Geometry: final body of the model. Coordinates: model frame, mm. Give positions to 0.01 mm unless a question says otherwise; leave off trailing zeros. Write each loop counter-clockwise with the first axis right and the second up, starting at its lowest first coordinate (ties: lowest second). Pieces come first, ordered by that corner, then holes. Notation, with made-up numbers: M 49.25,-1 L 79.25,-1 A18 ccw 79.25,27 Z; hole C -12.75,15 d8. An arc over 180 degrees is marked long. Answer as a JSON object with one key per item and string values.
from build123d import *

# Parameters (mm, degrees)
ESQUISSE1_R        = 75
ESQUISSE1_R_2      = 0.8
ESQUISSE1_R_3      = 3
ESQUISSE1_R_4      = 2
BOSS_EXTRU_1_DEPTH = 10


with BuildPart() as part:
    # Esquisse1 → Boss.-Extru.1 (new body)
    with BuildSketch(Plane(origin=(0, 0, 0), x_dir=(1, 0, 0), z_dir=(0, 1, 0))):
        with Locations(Location((0, 0, 0), (0, 0, 270))):
            Circle(ESQUISSE1_R)
        with Locations(Location((0, -7.5, 0), (0, 0, 270))):
            Circle(ESQUISSE1_R_2, mode=Mode.SUBTRACT)
        with Locations(Location((-7.5, 0, 0), (0, 0, 270))):
            Circle(ESQUISSE1_R_2, mode=Mode.SUBTRACT)
        with Locations(Location((0, 7.5, 0), (0, 0, 270))):
            Circle(ESQUISSE1_R_2, mode=Mode.SUBTRACT)
        with Locations(Location((7.5, 0, 0), (0, 0, 270))):
            Circle(ESQUISSE1_R_2, mode=Mode.SUBTRACT)
        with Locations(Location((0, 0, 0), (0, 0, 270))):
            Circle(ESQUISSE1_R_3, mode=Mode.SUBTRACT)
        with Locations(Location((0, 65, 0), (0, 0, 270))):
            Circle(ESQUISSE1_R_4, mode=Mode.SUBTRACT)
        with Locations(Location((0, -65, 0), (0, 0, 270))):
            Circle(ESQUISSE1_R_4, mode=Mode.SUBTRACT)
    extrude(amount=BOSS_EXTRU_1_DEPTH)


solid = part.part
1) Cut plane A-A on y = 4.5. Return loops of the section in (x, z), and give its area (3 significant figures).
Geometry check:
{"outline": "C 0,0 d150; hole C -7.5,0 d1.6; hole C 0,0 d6; hole C 0,-65 d4; hole C 0,65 d4; hole C 0,-7.5 d1.6; hole C 0,7.5 d1.6; hole C 7.5,0 d1.6", "area": "17,600 mm2"}
2) Cut plane B-B on z = 65. Return loops of the section in (x, y).
Geometry check:
{"outline": "M -37.42,0 L -2,0 L -2,10 L -37.42,10 Z; M 2,0 L 37.42,0 L 37.42,10 L 2,10 Z"}
3) Cut plane D-D on z = 40. Return loops of the section in (x, y).
Geometry check:
{"outline": "M -63.44,0 L 63.44,0 L 63.44,10 L -63.44,10 Z"}
4) Pull-direction query (Z, two-part tool) for faces 1 (the cylindrical face through (-45.636, 4.93, -59.517)), 2 (the flat face through (-16, 10, -1)), 3 (the cylindrical face through (0.9, 4.93, 2.86)); classes: pulls with the +Z half, pulls with the -Z half, needs draft (parallel to the pull), parting line crosses it, or undercut.
Geometry check:
{"face 1": "parting line crosses it", "face 2": "needs draft", "face 3": "undercut"}
5) Cut plane C-C on x = -23. Return loops of the section in (y, z).
Geometry check:
{"outline": "M 0,-71.39 L 10,-71.39 L 10,71.39 L 0,71.39 Z"}
6) Line query: line 1 (X direction, y = 2.5, z = 0); line 2 (Z direction, x = -1, y = 3.5); line 3 (X direction, y = 4.25, z = 7.5). Output: solid intervals per line, ascending. Write a range as from..to.
Geometry check:
{"line 1": "x = -75..-8.3, -6.7..-3, 3..6.7, 8.3..75", "line 2": "z = -74.99..-66.73, -63.27..-2.83, 2.83..63.27, 66.73..74.99", "line 3": "x = -74.62..-0.8, 0.8..74.62"}
7) Contact query for flat-ended pins moving along their axis: P1, Ø2, axis at x = 7.5, z = 0, coming from the +Y side; P2, Ø5, axis at y = 7.5, z = -26, coming from the +X side; P3, Ø1, axis at x = 6, y = 1, coming from the +Z side. Output: stop coordinate, or through.
Geometry check:
{"P1": "stops at y = 10", "P2": "stops at x = 71.22", "P3": "stops at z = 74.8"}
